For this review, take the finished solid that the model builds, in its own axes (mm). Face numbers are marked on the shaded views. A direction names the side the tool comes from. Coordinates: 2 decimals unless noted, no trailing zeros. Loops run counter-clockwise (first coordinate to the right, second up) from the corner with the lowest first, then second, coordinate; pieces in that order, holes last. Notation, with made-up numbers: (39, 55.25) - (90, 55.25) arc R22 ccw to (90, 72.25) - close; hole circle Ø3 at (0.5, 1). An arc over 180 degrees is marked (long way). Answer as a JSON object with one key per item and string values. Group by question number.
Item 1: To check wall thickness, follow line 1 (X direction, y = 12, z = 0); line 2 (X direction, y = 6.5, z = 0); line 3 (X direction, y = 10.5, z = -12). State the ranges of each line that lie inside material, in increasing order.
Item 2: We need section A-A (y = -0.5). State how many separate pieces and enclosed holes the cut face has, then the cut area to 3 significant figures.
Item 3: Mouldability with a two-part tool opening along X and no side actions: class the marked faces 1, 2 and 3 as released by +X, released by -X, zero draft, split by the parting line, or undercut.
Item 4: We need section D-D (z = -7). Give the boundary of the cut face in (x, y).
Item 5: Clearance check with flat-ended pins moving along their axes: pin 1 (5 mm diameter, centred on x = 63, z = 0.5, fed in from +Y); pin 2 (12 mm diameter, centred on x = 41.5, z = 1.5, fed in from +Y); pin 3 (12.5 mm diameter, centred on y = 17.5, z = 6.5, fed in from -X). State where each tip first meets the part, or that it passes through.
Item 6: Tool access review of the marked faces 4, 5, 6 and 7: name each direction out of +Z, -Z, +X, -X, +Y, -Y from which nothing blocks a thin tool from reaching the whole face with its end or side.
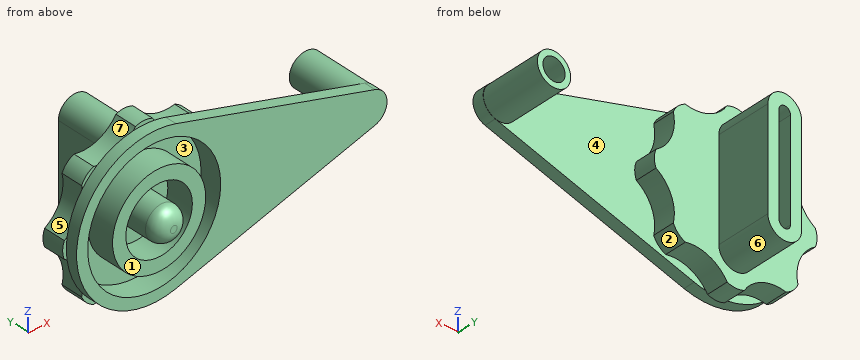
from build123d import *

# Parameters (mm, degrees)
BOSS_EXTRUDE1_DEPTH = 1.651
BOSS_EXTRUDE2_DEPTH = 6.35
BOSS_EXTRUDE3_START = -6.35
BOSS_EXTRUDE3_DEPTH = 22.225
BOSS_EXTRUDE4_START = -1.5875
SKETCH5_R           = 4.7625
BOSS_EXTRUDE4_DEPTH = 19.05
SKETCH6_R           = 3.175
CUT_EXTRUDE1_DEPTH  = 17.4625
SKETCH7_R           = 19.05
CUT_EXTRUDE3_DEPTH  = 6.35
SKETCH8_R           = 13.335
SKETCH8_R_2         = 9.525
BOSS_EXTRUDE5_DEPTH = 7.9375
SKETCH9_R           = 4.7625
BOSS_EXTRUDE6_DEPTH = 12.7
FILLET3_R           = 3.81


with BuildPart() as part:
    # Sketch1 → Boss-Extrude1 (new body, symmetric)
    with BuildSketch(Plane(origin=(0, 0, 0), x_dir=(1, 0, 0), z_dir=(0, 1, 0))):
        with BuildLine():
            Line((6.252207392, 21.327459477), (63.206622177, 4.631105486))
            ThreePointArc((63.206622177, 4.631105486), (66.675, 0), (63.206622177, -4.631105486))
            Line((63.206622177, -4.631105486), (6.252207392, -21.327459477))
            ThreePointArc((6.252207392, -21.327459477), (-22.225, 0), (6.252207392, 21.327459477))
        make_face()
    extrude(amount=BOSS_EXTRUDE1_DEPTH, both=True)

    # Sketch2 → Boss-Extrude2 (add)
    with BuildSketch(Plane(origin=(0, 1.651, 0), x_dir=(1, 0, 0), z_dir=(0, 1, 0))):
        with BuildLine():
            ThreePointArc((-17.844535667, 14.407940431), (-16.468028697, 16.468028697), (-14.407940431, 17.844535667))
            ThreePointArc((-14.407940431, 17.844535667), (-7.620469402, 18.397440581), (-2.430039796, 22.80594456))
            ThreePointArc((-2.430039796, 22.80594456), (0, 23.289309528), (2.430039796, 22.80594456))
            ThreePointArc((2.430039796, 22.80594456), (7.620469402, 18.397440581), (14.407940431, 17.844535667))
            ThreePointArc((14.407940431, 17.844535667), (16.468028697, 16.468028697), (17.844535667, 14.407940431))
            ThreePointArc((17.844535667, 14.407940431), (18.397440581, 7.620469402), (22.80594456, 2.430039796))
            ThreePointArc((22.80594456, 2.430039796), (23.289309528, 0), (22.80594456, -2.430039796))
            ThreePointArc((22.80594456, -2.430039796), (18.397440581, -7.620469402), (17.844535667, -14.407940431))
            ThreePointArc((17.844535667, -14.407940431), (16.468028697, -16.468028697), (14.407940431, -17.844535667))
            ThreePointArc((14.407940431, -17.844535667), (7.620469402, -18.397440581), (2.430039796, -22.80594456))
            ThreePointArc((2.430039796, -22.80594456), (0, -23.289309528), (-2.430039796, -22.80594456))
            ThreePointArc((-2.430039796, -22.80594456), (-7.620469402, -18.397440581), (-14.407940431, -17.844535667))
            ThreePointArc((-14.407940431, -17.844535667), (-16.468028697, -16.468028697), (-17.844535667, -14.407940431))
            ThreePointArc((-17.844535667, -14.407940431), (-18.397440581, -7.620469402), (-22.80594456, -2.430039796))
            ThreePointArc((-22.80594456, -2.430039796), (-23.289309528, 0), (-22.80594456, 2.430039796))
            ThreePointArc((-22.80594456, 2.430039796), (-18.397440581, 7.620469402), (-17.844535667, 14.407940431))
        make_face()
    extrude(amount=BOSS_EXTRUDE2_DEPTH)

    # Sketch4 → Boss-Extrude3 (add)
    with BuildSketch(Plane(origin=(0, 8.001, 0), x_dir=(1, 0, 0), z_dir=(0, 1, 0)).offset(BOSS_EXTRUDE3_START)):
        with BuildLine():
            Line((-4.826, -14.224), (-4.826, 14.224))
            ThreePointArc((-4.826, 14.224), (0, 19.05), (4.826, 14.224))
            Line((4.826, 14.224), (4.826, -14.224))
            ThreePointArc((4.826, -14.224), (0, -19.05), (-4.826, -14.224))
        make_face()
        with BuildLine():
            Line((-1.651, -14.224), (-1.651, 14.224))
            ThreePointArc((-1.651, 14.224), (0, 15.875), (1.651, 14.224))
            Line((1.651, 14.224), (1.651, -14.224))
            ThreePointArc((1.651, -14.224), (0, -15.875), (-1.651, -14.224))
        make_face(mode=Mode.SUBTRACT)
    extrude(amount=BOSS_EXTRUDE3_DEPTH)

    # Sketch5 → Boss-Extrude4 (add)
    with BuildSketch(Plane(origin=(0, 1.651, 0), x_dir=(1, 0, 0), z_dir=(0, 1, 0)).offset(BOSS_EXTRUDE4_START)):
        with Locations((61.849, 0)):
            Circle(SKETCH5_R)
    extrude(amount=BOSS_EXTRUDE4_DEPTH)

    # Sketch6 → Cut-Extrude1 (cut)
    with BuildSketch(Plane(origin=(0, 19.1135, 0), x_dir=(1, 0, 0), z_dir=(0, 1, 0))):
        with Locations((61.849, 0)):
            Circle(SKETCH6_R)
    extrude(amount=-CUT_EXTRUDE1_DEPTH, mode=Mode.SUBTRACT)

    # Sketch7 → Cut-Extrude3 (cut)
    with BuildSketch(Plane(origin=(0, -1.651, 0), x_dir=(1, 0, 0), z_dir=(0, 1, 0))):
        Circle(SKETCH7_R)
    extrude(amount=CUT_EXTRUDE3_DEPTH, mode=Mode.SUBTRACT)

    # Sketch8 → Boss-Extrude5 (add)
    with BuildSketch(Plane.XZ.offset(-4.699)):
        Circle(SKETCH8_R)
        Circle(SKETCH8_R_2, mode=Mode.SUBTRACT)
    extrude(amount=BOSS_EXTRUDE5_DEPTH)

    # Sketch9 → Boss-Extrude6 (add)
    with BuildSketch(Plane.XZ.offset(-4.699)):
        Circle(SKETCH9_R)
    extrude(amount=BOSS_EXTRUDE6_DEPTH)

    # Fillet3
    fillet3_edges = [part.edges().sort_by_distance(p)[0] for p in [
        (-4.7625, -8.001, 0),
    ]]
    fillet(fillet3_edges, radius=FILLET3_R)


solid = part.part
Check sheet entries:
{
 "1": {"line 1": "x = -4.83 to -1.65, 1.65 to 4.83, 57.09 to 58.67, 65.02 to 66.61", "line 2": "x = -23.29 to 23.29, 57.09 to 58.67, 65.02 to 66.61", "line 3": "x = -4.83 to -1.65, 1.65 to 4.83"},
 "2": {"separate pieces": "3", "enclosed holes": "2", "area": "1,760 mm2"},
 "3": {"face 1": "zero draft", "face 2": "released by +X", "face 3": "undercut"},
 "4": {"outline": "(-21.09, -1.65) - (-17.72, -1.65) - (-17.72, 4.7) - (-11.35, 4.7) - (-11.35, -3.24) - (-6.46, -3.24) - (-6.46, 4.7) - (6.46, 4.7) - (6.46, -3.24) - (11.35, -3.24) - (11.35, 4.7) - (17.72, 4.7) - (17.72, -1.65) - (55.13, -1.65) - (55.13, 1.65) - (18.68, 1.65) - (18.68, 8) - (4.83, 8) - (4.83, 23.88) - (1.65, 23.88) - (1.65, 8) - (-1.65, 8) - (-1.65, 23.88) - (-4.83, 23.88) - (-4.83, 8) - (-18.68, 8) - (-18.68, 1.65) - (-21.09, 1.65) - close"},
 "5": {"pin 1": "stops at y = 19.11", "pin 2": "stops at y = 1.65", "pin 3": "stops at x = -4.83"},
 "6": {"face 4": "+Y", "face 5": "-X, +Y", "face 6": "-Z, +Y", "face 7": "+Z, +Y"}
}
